Read the model definition and answer for the solid it produces. Units are mm, in the model's axes. A direction names the side the tool comes from. Give positions to 0.01 mm unless a question says otherwise; leave off trailing zeros. Loops run counter-clockwise (first coordinate to the right, second up) from the corner with the lowest first, then second, coordinate; pieces in that order, holes last. Notation, with made-up numbers: (42.25, 6) -> (69.25, 6) arc R16 cw to (69.25, 10) -> close; hole circle Ø4 at (-21, -26). An arc over 180 degrees is marked (long way). Write each question's results on one line, items separated by ' | '. Start each with the question number.
Item 1: Determine the mould class of faces 1 (the cylindrical face through (-10.124, 0.493, -2.249)), 2 (the flat face through (10, 0.5, -3.7)), 3 (the flat face through (2.5, 0.5, -2.3)) for opening direction Z: +Z half, -Z half, draft (parallel to the pull), parting line (faces both ways), or undercut.
Item 2: Section B-B on y = 0.45 is taken. Write down the section's boundary in (x, z) (1 decimal), and give its area (3 significant figures).
Item 3: Each of these flat-tipped pins is pushed along its axis until it touches: P1, Ø1.5, axis at x = -19.5, z = 15, coming from the -Y side; P2, Ø0.5, axis at x = 1, y = 0.5, coming from the +Z side. Where does it stop, or does it pass through?
Item 4: Section D-D on x = -13.5 is taken. Write down the section's boundary in (y, z), and give its area (3 significant figures).
Item 5: Section A-A on x = -3 is taken. Write down the section's boundary in (y, z).
Item 6: Find the intervals of material crossed by line 1 (Z direction, x = 6, y = 0.15); line 2 (X direction, y = 0.8, z = -3); line 3 (X direction, y = 0.1, z = -2.75), in increasing order.
Item 7: Section C-C on z = -1.25 is taken. Write down the section's boundary in (x, y), and give its area (3 significant figures).
Item 8: Which of the six approach directions +Z, -Z, +X, -X, +Y, -Y give full straight-line access (tool end or side, diameter ignored) to faces 4 (the flat face through (-27.539, 0.5, 15.7)), 5 (the flat face through (-0.4, 0.5, 5)), 6 (the flat face through (-10, 0.5, -3.5)), 7 (the flat face through (2.7, 0.5, 2.3))?
```python
from build123d import *

# Parameters (mm, degrees)
BOSS_EXTRUDE1_DEPTH   = 1
CUT_EXTRUDE1_DEPTH    = 2
FILLET1_R             = 0.79375
CHAMFER1_SIZE         = 0.79375
CHAMFER1_EDGE_2_SIZE  = 0.79375
CHAMFER1_EDGE_3_SIZE  = 0.619288519
CHAMFER1_EDGE_3_SIZE2 = 0.79375
CHAMFER1_EDGE_4_SIZE  = 0.79375
CHAMFER1_EDGE_5_SIZE  = 0.79375


with BuildPart() as part:
    # Sketch1 → Boss-Extrude1 (new body)
    with BuildSketch(Plane(origin=(0, 0, 0), x_dir=(1, 0, 0), z_dir=(0, 1, 0))):
        with BuildLine():
            Line((-11.680023612, -5.916593509), (-18.433746975, -20.4))
            Line((-18.433746975, -20.4), (-28.1, -15.892552189))
            Line((-28.1, -15.892552189), (-10.464967985, 1.742479827))
            ThreePointArc((-10.464967985, 1.742479827), (-10.120841242, 2.257501893), (-10, 2.865011842))
            Line((-10, 2.865011842), (-10, 5))
            Line((-10, 5), (10, 5))
            Line((10, 5), (10, -5))
            Line((10, -5), (-10.24126, -5))
            ThreePointArc((-10.24126, -5), (-11.094223128, -5.24861608), (-11.680023612, -5.916593509))
        make_face()
    extrude(amount=BOSS_EXTRUDE1_DEPTH)

    # Sketch2 → Cut-Extrude1 (cut, through all)
    with BuildSketch(Plane(origin=(0, 1, 0), x_dir=(1, 0, 0), z_dir=(0, 1, 0))):
        with BuildLine():
            Line((-3.99999994, 2.3), (10, 2.3))
            Line((10, 2.3), (10, -2.3))
            Line((10, -2.3), (-3.99999994, -2.3))
            ThreePointArc((-3.99999994, -2.3), (-6.29999994, 0), (-3.99999994, 2.3))
        make_face()
    extrude(amount=-CUT_EXTRUDE1_DEPTH, mode=Mode.SUBTRACT)

    # Fillet1
    fillet1_edges = [part.edges().sort_by_distance(p)[0] for p in [
        (10, 0.5, -2.3),
        (10, 0.5, 2.3),
    ]]
    fillet(fillet1_edges, radius=FILLET1_R)

    # Chamfer1
    chamfer1_edges = [part.edges().sort_by_distance(p)[0] for p in [
        (10, 0.5, 5),
    ]]
    chamfer(chamfer1_edges, length=CHAMFER1_SIZE)

    # Chamfer1 edge 2
    chamfer1_edge_2_edges = [part.edges().sort_by_distance(p)[0] for p in [
        (-18.433746975, 0.5, 20.4),
    ]]
    chamfer(chamfer1_edge_2_edges, length=CHAMFER1_EDGE_2_SIZE)

    # Chamfer1 edge 3
    chamfer1_edge_3_edges = [part.edges().sort_by_distance(p)[0] for p in [
        (-28.1, 0.5, 15.892552189),
    ]]
    chamfer1_edge_3_side = [part.faces().sort_by_distance(p)[0] for p in [
        (-23.266873487, 0.5, 18.146276094),
    ]]
    chamfer(chamfer1_edge_3_edges, length=CHAMFER1_EDGE_3_SIZE, length2=CHAMFER1_EDGE_3_SIZE2, reference=chamfer1_edge_3_side[0])

    # Chamfer1 edge 4
    chamfer1_edge_4_edges = [part.edges().sort_by_distance(p)[0] for p in [
        (-10, 0.5, -5),
    ]]
    chamfer(chamfer1_edge_4_edges, length=CHAMFER1_EDGE_4_SIZE)

    # Chamfer1 edge 5
    chamfer1_edge_5_edges = [part.edges().sort_by_distance(p)[0] for p in [
        (10, 0.5, -5),
    ]]
    chamfer(chamfer1_edge_5_edges, length=CHAMFER1_EDGE_5_SIZE)


solid = part.part
```
Findings:
1) face 1: -Z half | face 2: draft | face 3: undercut
2) outline: (-27.5, 15.3) -> (-10.5, -1.7) arc R1.6 cw to (-10, -2.9) -> (-10, -4.2) -> (-9.2, -5) -> (9.2, -5) -> (10, -4.2) -> (10, -3.1) arc R0.8 ccw to (9.2, -2.3) -> (-4, -2.3) arc R2.3 cw to (-4, 2.3) -> (9.2, 2.3) arc R0.8 ccw to (10, 3.1) -> (10, 4.2) -> (9.2, 5) -> (-10.2, 5) arc R1.6 cw to (-11.7, 5.9) -> (-18.1, 19.7) -> (-19.2, 20.1) -> (-27.5, 16.2) -> close | area: 275 mm2
3) P1: y = 0 | P2: z = 5
4) outline: (0, 1.29) -> (1, 1.29) -> (1, 9.82) -> (0, 9.82) -> close | area: 8.53 mm2
5) outline: (0, -5) -> (1, -5) -> (1, -2.3) -> (0, -2.3) -> close; (0, 2.3) -> (1, 2.3) -> (1, 5) -> (0, 5) -> close
6) line 1: -5 to -2.3, 2.3 to 5 | line 2: -10 to 9.99 | line 3: -10 to 9.92
7) outline: (-10.96, 0) -> (-5.93, 0) -> (-5.93, 1) -> (-10.96, 1) -> close | area: 5.03 mm2
8) face 4: +Z, -Z, -X, +Y, -Y | face 5: +Z, +X, +Y, -Y | face 6: -Z, -X, +Y, -Y | face 7: +X, +Y, -Y
